Here's how the part is built. I have some questions about the finished solid (model axes, mm). Face numbers are marked on the shaded views. A direction names the side the tool comes from. Round coordinates to 2 decimals unless told otherwise and drop trailing zeros. Loops run counter-clockwise (first coordinate to the right, second up) from the corner with the lowest first, then second, coordinate; pieces in that order, holes last. Notation, with made-up numbers: M -39,80.5 L 17,80.5 A31 ccw 17,109.5 Z; hole C -38.5,70 d11. An arc over 180 degrees is marked long. Write each question's results on one line, items separated by ' | '. Start each with the question number.
```python
from build123d import *

# Parameters (mm, degrees)
F1_DEPTH = 2
F3_DEPTH = 25


with BuildPart() as f1:
    # F0 (on Top) → F1 (new body)
    with BuildSketch(Plane.XY):
        with BuildLine():
            Line((0, 55), (0, 0))
            Line((0, 0), (120, 0))
            Line((120, 0), (120, 55))
            ThreePointArc((120, 55), (118.535534, 58.535534), (115, 60))
            Line((115, 60), (5, 60))
            ThreePointArc((5, 60), (1.464466, 58.535534), (0, 55))
        make_face()
    extrude(amount=F1_DEPTH)

    # F2 (on face) → F3 (join)
    with BuildSketch(Plane.XY.offset(2)):
        with BuildLine():
            Line((0, 55), (0, 0))
            Line((0, 0), (1.5, 0))
            Line((1.5, 0), (1.5, 55))
            ThreePointArc((1.5, 55), (2.525126, 57.474874), (5, 58.5))
            Line((5, 58.5), (115, 58.5))
            ThreePointArc((115, 58.5), (117.474874, 57.474874), (118.5, 55))
            Line((118.5, 55), (118.5, 0))
            Line((118.5, 0), (120, 0))
            Line((120, 0), (120, 55))
            ThreePointArc((120, 55), (118.535534, 58.535534), (115, 60))
            Line((115, 60), (5, 60))
            ThreePointArc((5, 60), (1.464466, 58.535534), (0, 55))
        make_face()
    extrude(amount=F3_DEPTH)


solid = f1.part
```
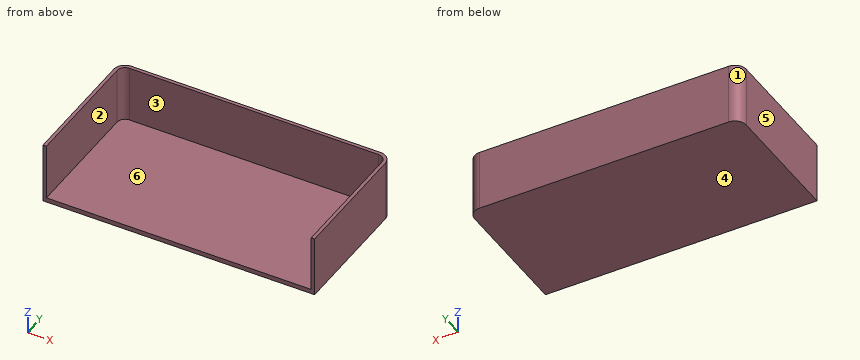
Item 1: I need wall thicknesses on L1, parallel to X at y = 40, z = 13.5; L2, parallel to Y at x = 60, z = 8.25; L3, parallel to Z at x = 112.5, y = 36.5. Which ranges of each line are inside material? Lowest first, please.
Item 2: I'm going to push flat-ended pins straight in: pin 1 (17.5 mm diameter, centred on x = 86, y = 14.5, fed in from +Z); pin 2 (4 mm diameter, centred on x = 16, z = 9, fed in from -Y). Where does each tip first touch, or does it pass through?
Item 3: If we section it at C-C on z = 10: Please give me the cut outline in (x, y).
Item 4: If we section it at A-A on y = 21.5: Please give me the cut outline in (x, z), and give its area (3 significant figures).
Item 5: If we mould it in two halves opening along X, with no side actions, what happens to the marked faces 1, 2, 3 and 4? For each: released by +X, released by -X, zero draft, split by the parting line, or undercut.
Item 6: Which directions (+Z, -Z, +X, -X, +Y, -Y) give clear straight access to the entire face, cutting with the end or side of a thin tool? Please do the marked faces 5 and 6.
Item 7: If we section it at B-B on x = 109: Please give me the cut outline in (y, z).
Numbers:
1) L1: 0 to 1.5, 118.5 to 120 | L2: 58.5 to 60 | L3: 0 to 2
2) pin 1: z = 2 | pin 2: y = 58.5
3) outline: M 0,0 L 1.5,0 L 1.5,55 A3.5 cw 5,58.5 L 115,58.5 A3.5 cw 118.5,55 L 118.5,0 L 120,0 L 120,55 A5 ccw 115,60 L 5,60 A5 ccw 0,55 Z
4) outline: M 0,0 L 120,0 L 120,27 L 118.5,27 L 118.5,2 L 1.5,2 L 1.5,27 L 0,27 Z | area: 315 mm²
5) face 1: released by -X | face 2: undercut | face 3: undercut | face 4: zero draft
6) face 5: +Z, -Z, -X, +Y, -Y | face 6: +Z, -Y
7) outline: M 0,0 L 60,0 L 60,27 L 58.5,27 L 58.5,2 L 0,2 Z
